The listing builds one solid part. Answer for the finished solid, in the listing's coordinates (mm). Give positions to 0.01 mm unless a question says otherwise; leave off trailing zeros. Order: outer loops, then holes, each group sorted by start corner. A loop starts at its lowest first (then second) coordinate and runs counter-clockwise, first axis right, second up. Notation, with made-up numbers: (-32, 78.25) - (21, 78.25) arc R23 ccw to (21, 111.25) - close; hole circle Ø3 at (-3, 25). An arc over 180 degrees is marked (long way). Answer in a Markdown table with one row per item.
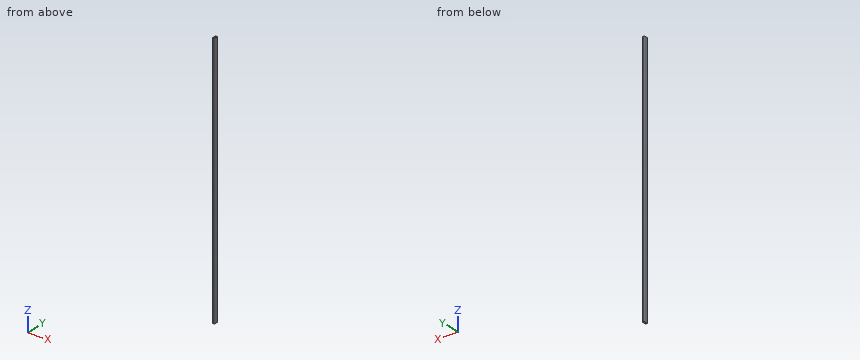
Autodesk Inventor part; units mm, degrees
ref_plane "Start plane" through (0, 0, 0) normal (0, 0, 1) x (1, 0, 0)
ref_plane "End plane" through (0, 0, 2600) normal (0, 0, 1) x (1, 0, 0)
ref_plane "YZ Plane" through (0, 0, 0) normal (1, 0, 0) x (0, 1, 0)
ref_plane "Start plane" through (0, 0, 0) normal (0, 0, 1) x (1, 0, 0)
ref_plane "End plane" through (0, 0, 2600) normal (0, 0, 1) x (1, 0, 0)
sketch "Sketch" plane through (0, 0, 0) normal (0, 0, 1) x (1, 0, 0)
  line L0 (-10, -16) -> (-10, 16)
  line L1 (-6, 20) -> (6, 20)
  line L2 (10, 16) -> (10, -16)
  line L3 (6, -20) -> (-6, -20)
  arc A0 (-10, -16) -> (-6, -20) centre (-6, -16) ccw
  arc A1 (10, 16) -> (6, 20) centre (6, 16) ccw
  arc A2 (-6, 20) -> (-10, 16) centre (-6, 16) ccw
  arc A3 (6, -20) -> (10, -16) centre (6, -16) ccw
  arc A4 (-6, 18) -> (-8, 16) centre (-6, 16) ccw
  line L4 (-6, 18) -> (6, 18)
  arc A5 (8, 16) -> (6, 18) centre (6, 16) ccw
  line L5 (8, 16) -> (8, -16)
  arc A6 (6, -18) -> (8, -16) centre (6, -16) ccw
  line L6 (6, -18) -> (-6, -18)
  arc A7 (-8, -16) -> (-6, -18) centre (-6, -16) ccw
  line L7 (-8, -16) -> (-8, 16)
  line L8 (0, 37.1021) -> (0, -37.1021) construction
  line L9 (-23.1021, 0) -> (23.1021, 0) construction
  dimension "d7" = 4
  dimension "d9" = 20
  dimension "d11" = 40
  dimension "d12" = 2
  dimension "d15" = 10
  dimension "d16" = 20
extrude "Body" add sketch "Sketch" along normal up to surface (2600 mm away) from surface at 0
sketch "Sketch3" plane through (0, 0, 0) normal (0, 0, 1) x (1, 0, 0)
  line L0 (0, 0) -> (10, 0)
ref_plane "Work Plane3" through (0, 0, 0) normal (0, -1, 0) x (1, 0, 0)
ref_plane "Work Plane4" through (4294.7542, -381.1194, 3164.8652) normal (0, 1, 0) x (-1, 0, 0)
sketch "Sketch5" plane through (4294.7542, -381.1194, 3164.8652) normal (0, 1, 0) x (-1, 0, 0)
  point P0 (4294.7542, -3164.8652)
sketch "Sketch4" plane through (0, 0, 0) normal (0, -1, 0) x (1, 0, 0)
  line L0 (-2, 0) -> (12, 0)
  line L1 (-2, 2600) -> (12, 2600)
  dimension "d18" = 2600
equation "\"d7\" = G_IR"
equation "\"d9\" = G_W"
equation "\"d11\" = G_H"
equation "\"d12\" = G_T"
equation "\"d15\" = 0.5 * d9"
equation "\"d16\" = 0.5 * d11"
equation "\"d3\" = G_L"
equation "\"G_W\" = 20"
equation "\"G_H\" = 40"
equation "\"G_T\" = 2"
equation "\"G_IR\" = 4"
equation "\"G_L\" = d18"
equation "\"G_OFFSET_START\" = 0"
equation "\"G_OFFSET_END\" = 0"
properties part number "ISO 10799-2 - 40x20x2 - 2600" material "Steel, Mild"
Item 1: Find section C-C on z = 2274. Write down the section's boundary in (x, y), then the cut area to 3 significant figures.
Answer block:
| item | result |
|---|---|
| outline | (-10, -16) arc R4 ccw to (-6, -20) - (6, -20) arc R4 ccw to (10, -16) - (10, 16) arc R4 ccw to (6, 20) - (-6, 20) arc R4 ccw to (-10, 16) - close; hole (-8, -16) arc R2 ccw to (-6, -18) - (6, -18) arc R2 ccw to (8, -16) - (8, 16) arc R2 ccw to (6, 18) - (-6, 18) arc R2 ccw to (-8, 16) - close |
| area | 214 mm² |
Item 2: Consider line 1 (X direction, y = -3.5, z = 2480); line 2 (Y direction, x = 3.75, z = 964.5); line 3 (X direction, y = 16.5, z = 2309). Determine where each line is inside the solid, lowest interval first.
Answer block:
| item | result |
|---|---|
| line 1 | -10 to -8, 8 to 10 |
| line 2 | -20 to -18, 18 to 20 |
| line 3 | -9.97 to -7.94, 7.94 to 9.97 |
Item 3: Find section A-A on x = -3. Write down the section's boundary in (y, z), then the cut area to 3 significant figures.
Answer block:
| item | result |
|---|---|
| outline | (-20, 0) - (-18, 0) - (-18, 2600) - (-20, 2600) - close; (18, 0) - (20, 0) - (20, 2600) - (18, 2600) - close |
| area | 10,400 mm² |
Item 4: Find section B-B on y = 3.5. Write down the section's boundary in (x, z), then the cut area to 3 significant figures.
Answer block:
| item | result |
|---|---|
| outline | (-10, 0) - (-8, 0) - (-8, 2600) - (-10, 2600) - close; (8, 0) - (10, 0) - (10, 2600) - (8, 2600) - close |
| area | 10,400 mm² |
